Input: part model. Units: mm. Frame: model coordinates. Coordinates: 2 decimals unless noted, no trailing zeros. Write each loop counter-clockwise with the first axis right and the second up, starting at its lowest first coordinate (ties: lowest second). Pieces come first, ordered by that corner, then holes. Notation, with made-up numbers: M 21.25,18.25 L 50.25,18.25 A10 cw 50.25,24.25 Z; hole C 30,4 d9. An arc over 180 degrees is marked long. Use CSV: the item, a comma, the result in double quotes.
Autodesk Fusion 360 part; units mm, degrees
sketch "Sketch1" plane through (0, 0, 0) normal (0, 1, 0) x (1, 0, 0)
  line L0 (0, 0) -> (20, 0) construction
  line L1 (20, 0) -> (20, 24) construction
  line L2 (20, 24) -> (0, 24) construction
  line L3 (0, 24) -> (0, 0) construction
  circle A0 centre (0, 24) radius 1.1
  circle A1 centre (20, 24) radius 1.1
  circle A2 centre (20, 0) radius 1.1
  circle A3 centre (0, 0) radius 1.1
  line L4 (-2, 26) -> (22, 26)
  line L5 (22, 26) -> (22, -2)
  line L6 (22, -2) -> (-2, -2)
  line L7 (-2, -2) -> (-2, 26)
  line L8 (0, 24) -> (20, 24)
  line L9 (20, 24) -> (20, 0)
  line L10 (20, 0) -> (0, 0)
  line L11 (0, 0) -> (0, 24)
  dimension "d1" = 24
  dimension "d2" = 20
  dimension "d3" = 2.2
  dimension "d4" = 2
  dimension "d5" = 2
  dimension "d6" = 2
  dimension "d7" = 2
extrude "Extrude1" add sketch "Sketch1" along normal blind 2
fillet "Fillet1" radius 1 8 edges at (1.1, 1, -24) (0, 1, -22.9) (0, 1, -1.1) (18.9, 1, -24) (1.1, 1, 0) (20, 1, -22.9) (20, 1, -1.1) (18.9, 1, 0)
fillet "Fillet2" radius 1 4 edges at (-2, 1, -26) (-2, 1, 2) (22, 1, 2) (22, 1, -26)
extrude "Extrude2" cut 1 faces at (13.6667, 0.6667, 2) along direction (0, 0, -1) up to surface (2 mm away)
fillet "Fillet3" radius 0.4 2 edges at (-1, 1, 2) (21, 1, 2)
sketch "Sketch2" plane through (0, 2, 0) normal (0, 1, 0) x (-1, 0, 0)
  arc A0 (-21, 1.4472) -> (-21.6667, 1.7454) centre (-21.4, 1.4472) ccw
  arc A1 (-21.6667, 1.7454) -> (-22, 1) centre (-21, 1) ccw
  line L0 (-22, 1) -> (-22, -25)
  arc A2 (-22, -25) -> (-21, -26) centre (-21, -25) ccw
  line L1 (-21, -26) -> (1, -26)
  arc A3 (1, -26) -> (2, -25) centre (1, -25) ccw
  line L2 (2, -25) -> (2, 1)
  arc A4 (2, 1) -> (1.6667, 1.7454) centre (1, 1) ccw
  arc A5 (1.6667, 1.7454) -> (1, 1.4472) centre (1.4, 1.4472) ccw
  line L3 (1, 1.4472) -> (1, 0.4583)
  arc A6 (0.5238, -0.9673) -> (1, 0.4583) centre (0, 0) ccw
  arc A7 (0.5238, -0.9673) -> (0, -1.8466) centre (1, -1.8466) ccw
  line L4 (0, -1.8466) -> (0, -22.1534)
  arc A8 (0, -22.1534) -> (0.5238, -23.0327) centre (1, -22.1534) ccw
  arc A9 (-0.9673, -24.5238) -> (0.5238, -23.0327) centre (0, -24) ccw
  arc A10 (-0.9673, -24.5238) -> (-1.8466, -24) centre (-1.8466, -25) ccw
  line L5 (-1.8466, -24) -> (-18.1534, -24)
  arc A11 (-18.1534, -24) -> (-19.0327, -24.5238) centre (-18.1534, -25) ccw
  arc A12 (-20.5238, -23.0327) -> (-19.0327, -24.5238) centre (-20, -24) ccw
  arc A13 (-20.5238, -23.0327) -> (-20, -22.1534) centre (-21, -22.1534) ccw
  line L6 (-20, -22.1534) -> (-20, -1.8466)
  arc A14 (-20, -1.8466) -> (-20.5238, -0.9673) centre (-21, -1.8466) ccw
  arc A15 (-21, 0.4583) -> (-20.5238, -0.9673) centre (-20, 0) ccw
  line L7 (-21, 0.4583) -> (-21, 1.4472)
  line L8 (-3.4, -24) -> (-16.6, -24)
  line L9 (-16.6, -24) -> (-16.6, -25.4)
  line L10 (-16.6, -25.4) -> (-3.4, -25.4)
  line L11 (-3.4, -25.4) -> (-3.4, -24)
  line L12 (-1, -26) -> (-1, -27)
  line L13 (-1, -27) -> (-19, -27)
  line L14 (-19, -27) -> (-19, -26)
  line L15 (-1, -26) -> (-19, -26)
  dimension "d18" = 1.4
  dimension "d19" = 13.2
  dimension "d20" = 1
  dimension "d21" = 18
extrude "Extrude3" cut sketch "Sketch2" against normal up to surface (2 mm away) contours L5 L8 L9 L10 L11
extrude "Extrude4" add sketch "Sketch2" against normal up to surface (2 mm away) contours L1 L12 L13 L14 L15
fillet "Fillet5" radius 0.5 4 edges at (1, 1, -26) (1, 1, -27) (19, 1, -27) (19, 1, -26)
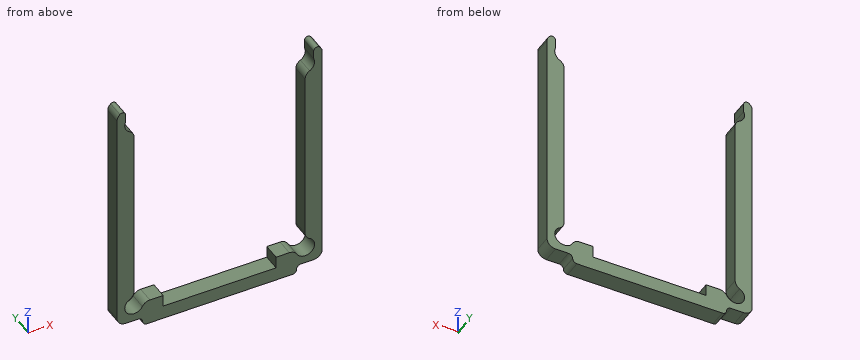
1. Section A-A (z = -19.25). Return loops of the section in (x, y), then the cut area to 3 significant figures.
Resolved:
outline,"M -2,0 L 0,0 L 0,2 L -2,2 Z; M 20,0 L 22,0 L 22,2 L 20,2 Z"
area,"8.00 mm^2"
2. Contact query for flat-ended pins moving along their axis: pin 1 Ø10 at (x, z) = (19, -24) entering from -Y; pin 2 Ø0.8 at (x, y) = (20.5, 1.5) entering from -Z; pin 3 Ø0.8 at (x, y) = (2.5, 0.5) entering from +Z. Output: stop coordinate, or through.
Resolved:
pin 1,"stops at y = 0"
pin 2,"stops at z = -26"
pin 3,"stops at z = -24"
3. Section B-B (x = 9.75). Return loops of the section in (y, z), then the cut area to 3 significant figures.
Resolved:
outline,"M 0,-27 L 2,-27 L 2,-25.4 L 0,-25.4 Z"
area,"3.20 mm^2"
4. Material intervals for line 1 (X direction, y = 0.6, z = -2); line 2 (Z direction, x = 14.5, y = 1.45); line 3 (X direction, y = 0.95, z = -0.25), sorted ascending. Write a range as [from, to].
Resolved:
line 1,"x = [-2, 0], [20, 22]"
line 2,"z = [-27, -25.4]"
line 3,"x = [-2, -1.07], [21.07, 22]"
